Source: CAD feature listing. Evaluate the final solid. Frame: model axes, mm. A direction names the side the tool comes from. Round coordinates to 2 decimals unless told otherwise and drop trailing zeros. Write each loop counter-clockwise with the first axis right and the second up, starting at its lowest first coordinate (ties: lowest second). Pieces come first, ordered by that corner, then holes. Notation, with made-up numbers: (-26.75, 46.25) - (25.25, 46.25) arc R35 cw to (25.25, 79.25) - close; hole circle Ø2 at (-30, 21.5). An arc over 180 degrees is marked (long way). Write item = value, one per line. Start each with the question number.
```python
from build123d import *

# Parameters (mm, degrees)
BOSS_EXTRUDE1_DEPTH = 15
SKETCH2_R           = 1.625
CUT_EXTRUDE1_DEPTH  = 6.25


with BuildPart() as part:
    # Sketch1 → Boss-Extrude1 (new body)
    with BuildSketch(Plane(origin=(0, 0, 0), x_dir=(0, 0, -1), z_dir=(1, 0, 0))):
        with BuildLine():
            Line((0, 4.25), (0, 0))
            Line((0, 0), (60, 0))
            Line((60, 0), (60, 6.25))
            Line((60, 6.25), (45, 6.25))
            Line((45, 6.25), (45, 2.25))
            Line((45, 2.25), (7, 2.25))
            Line((7, 2.25), (7, 4.25))
            ThreePointArc((7, 4.25), (6.414213562, 5.664213562), (5, 6.25))
            Line((5, 6.25), (2, 6.25))
            ThreePointArc((2, 6.25), (0.585786438, 5.664213562), (0, 4.25))
        make_face()
    extrude(amount=BOSS_EXTRUDE1_DEPTH)

    # Sketch2 → Cut-Extrude1 (cut)
    with BuildSketch(Plane.XZ):
        with Locations(Location((11, -52.5, 0), (0, 0, 270))):
            Circle(SKETCH2_R)
        with Locations(Location((4, -52.5, 0), (0, 0, 270))):
            Circle(SKETCH2_R)
    extrude(amount=-CUT_EXTRUDE1_DEPTH, mode=Mode.SUBTRACT)


solid = part.part
```
(1) Ray query, L1, parallel to X at y = 1.75, z = -52.5 (3 decimals); L2, parallel to Z at x = 10, y = 4.75; L3, parallel to Y at x = 2.5, z = -14. Return the intervals inside material, ascending. Write a range as from..to.
(2) Section D-D (y = 1.5). Return the cut outline in (x, z) (3 decimals).
(3) Section A-A (x = 4). Return the cut outline in (y, z) (3 decimals), plus the area to 3 significant figures.
(4) Contact query for a flat-ended pin moving along its axis: P1, Ø1.5, axis at x = 10.5, z = -14, coming from the +Y side. Output: stop coordinate, or through.
(5) Section C-C (y = 5.25). Return the cut outline in (x, z) (3 decimals), plus the area to 3 significant figures.
(6) Section B-B (z = -52.5). Return the cut outline in (x, y) (3 decimals), plus the area to 3 significant figures.
(7) Reachability of faces 4 (the flat face through (7, 6.25, -4)), 5 (the flat face through (7, 2.25, -26)) from +Z, -Z, +X, -X, +Y, -Y: full face, straight path, thin tool, end or side. Return the list, or none.
(8) Pull-direction query (X, two-part tool) for faces 1 (the cylindrical face through (4.071, 3.081, -50.877)), 2 (the flat face through (0, 2, -30)), 3 (the flat face through (7, 4, -45)); classes: +X half, -X half, draft (parallel to the pull), parting line (faces both ways), or undercut.
Solution:
q1.L1 = 0..2.375, 5.625..9.375, 12.625..15
q1.L2 = -60..-53.78, -51.22..-45, -6.94..-0.06
q1.L3 = 0..2.25
q2.outline = (0, -60) - (15, -60) - (15, 0) - (0, 0) - close; hole circle Ø3.25 at (4, -52.5); hole circle Ø3.25 at (11, -52.5)
q3.outline = (0, -60) - (6.25, -60) - (6.25, -54.125) - (0, -54.125) - close; (0, -50.875) - (6.25, -50.875) - (6.25, -45) - (2.25, -45) - (2.25, -7) - (4.25, -7) arc R2 ccw to (6.25, -5) - (6.25, -2) arc R2 ccw to (4.25, 0) - (0, 0) - close
q3.area = 201 mm^2
q4.P1 = 2.25
q5.outline = (0, -60) - (15, -60) - (15, -45) - (0, -45) - close; (0, -6.732) - (15, -6.732) - (15, -0.268) - (0, -0.268) - close; hole circle Ø3.25 at (4, -52.5); hole circle Ø3.25 at (11, -52.5)
q5.area = 305 mm^2
q6.outline = (0, 0) - (2.375, 0) - (2.375, 6.25) - (0, 6.25) - close; (5.625, 0) - (9.375, 0) - (9.375, 6.25) - (5.625, 6.25) - close; (12.625, 0) - (15, 0) - (15, 6.25) - (12.625, 6.25) - close
q6.area = 53.1 mm^2
q7.face_4 = +Z, -Z, +X, -X, +Y
q7.face_5 = +X, -X, +Y
q8.face_1 = undercut
q8.face_2 = -X half
q8.face_3 = draft
